Read the model definition and answer for the solid it produces. Units are mm, in the model's axes. Face numbers are marked on the shaded views. A direction names the side the tool comes from. Give positions to 0.01 mm unless a question says otherwise; leave off trailing zeros. Write each loop counter-clockwise with the first axis right and the second up, starting at its lowest first coordinate (ties: lowest second). Pieces come first, ordered by that corner, then holes. Notation, with made-up numbers: M 51,-1 L 97,-1 A19 cw 97,35 Z; hole C 20,-21.75 d8. An arc over 180 degrees is marked long. Put each result on its own line as item: value.
from build123d import *

# Parameters (mm, degrees)
F0_R     = 28.575
F1_DEPTH = 12.7
F2_R     = 15.875
F3_DEPTH = 12.7
F4_R     = 9.525
F5_DEPTH = 25.401
F6_R     = 3.175
F7_DEPTH = 12.701


with BuildPart() as f1:
    # F0 (on Top) → F1 (new body)
    with BuildSketch(Plane.XY):
        Circle(F0_R)
    extrude(amount=F1_DEPTH)

    # F2 (on face) → F3 (join)
    with BuildSketch(Plane.XY.offset(12.7)):
        Circle(F2_R)
    extrude(amount=F3_DEPTH)

    # F4 (on face) → F5 (cut, through all)
    with BuildSketch(Plane.XY.offset(25.4)):
        Circle(F4_R)
    extrude(amount=-F5_DEPTH, mode=Mode.SUBTRACT)

    # F6 (on face) → F7 (cut, through all)
    with BuildSketch(Plane.XY.offset(12.7)):
        with Locations((0, 22.225)):
            Circle(F6_R)
        with Locations((22.225, 0)):
            Circle(F6_R)
        with Locations((-22.225, 0)):
            Circle(F6_R)
        with Locations((0, -22.225)):
            Circle(F6_R)
    extrude(amount=-F7_DEPTH, mode=Mode.SUBTRACT)


solid = f1.part
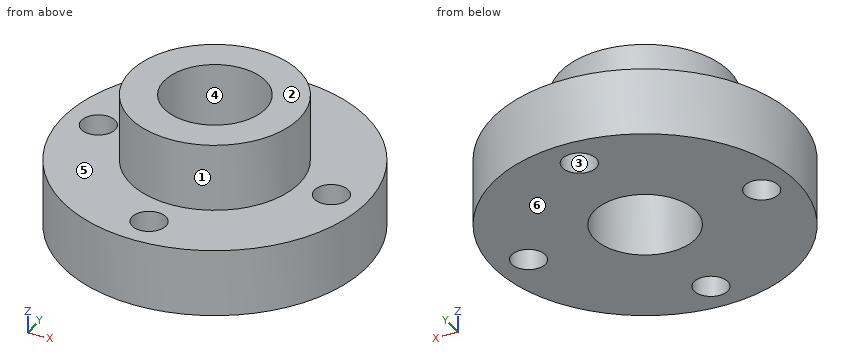
(1) Straight lines are drawn through the part: line 1 along Y through (x, z) = (0, 6.5) (3 decimals); line 2 along Y through (x, z) = (0, 16.25) (3 decimals); line 3 along X through (y, z) = (1, 9.5). For each, find the intervals that lie inside material, in ascending order. Write a range as from..to.
Result:
line 1: y = -28.575..-25.4, -19.05..-9.525, 9.525..19.05, 25.4..28.575
line 2: y = -15.875..-9.525, 9.525..15.875
line 3: x = -28.56..-25.24, -19.21..-9.47, 9.47..19.21, 25.24..28.56
(2) Which of the six approach directions +Z, -Z, +X, -X, +Y, -Y give full straight-line access (tool end or side, diameter ignored) to the marked faces 5 and 6?
Result:
face 5: +Z
face 6: -Z, +X, -X, +Y, -Y
(3) Section D-D on z = 20.25 is taken. Determine the outline of the cut face in (x, y) (3 decimals), and give its area (3 significant figures).
Result:
outline: C 0,0 d31.75; hole C 0,0 d19.05
area: 507 mm²
(4) Section C-C on x = -8 is taken. Determine the outline of the cut face in (y, z), and give its area (3 significant figures).
Result:
outline: M -27.43,0 L -5.17,0 L -5.17,25.4 L -13.71,25.4 L -13.71,12.7 L -27.43,12.7 Z; M 5.17,0 L 27.43,0 L 27.43,12.7 L 13.71,12.7 L 13.71,25.4 L 5.17,25.4 Z
area: 782 mm²
(5) For a pull along X with two mould halves and no side action, classify the marked faces 1, 2, 3 and 4 as +X half, -X half, draft (parallel to the pull), parting line (faces both ways), or undercut.
Result:
face 1: parting line
face 2: draft
face 3: undercut
face 4: undercut
(6) Section A-A on x = 0 is taken. Determine the outline of the cut face in (y, z) (3 decimals), and give its area (3 significant figures).
Result:
outline: M -28.575,0 L -25.4,0 L -25.4,12.7 L -28.575,12.7 Z; M -19.05,0 L -9.525,0 L -9.525,25.4 L -15.875,25.4 L -15.875,12.7 L -19.05,12.7 Z; M 9.525,0 L 19.05,0 L 19.05,12.7 L 15.875,12.7 L 15.875,25.4 L 9.525,25.4 Z; M 25.4,0 L 28.575,0 L 28.575,12.7 L 25.4,12.7 Z
area: 484 mm²
(7) Given pin 1 Ø5 at (y, z) = (-14.5, 5) entering from +X; pin 2 Ø7.5 at (x, y) = (0, -22.225) entering from +Z; pin 3 Ø1 at (y, z) = (-9, 15.5) entering from -X, each flat-ended and moving along its own axis, determine where each tip first touches the part or whether it passes through.
Result:
pin 1: stops at x = 25.93
pin 2: stops at z = 12.7
pin 3: stops at x = -13.41
